Autodesk Inventor part; units mm, degrees
ref_plane "YZ Plane" through (0, 0, 0) normal (1, 0, 0) x (0, 1, 0)
ref_plane "XZ Plane" through (0, 0, 0) normal (0, 1, 0) x (-1, 0, 0)
ref_plane "XY Plane" through (0, 0, 0) normal (0, 0, 1) x (1, 0, 0)
sketch "スケッチ1" plane through (0, 0, 0) normal (0, 0, 1) x (1, 0, 0)
  circle A0 centre (0, 0) radius 23
  dimension "d0" = 46
extrude "押し出し1" add sketch "スケッチ1" along normal blind 6.3
sketch "スケッチ2" plane through (0, 0, 6.3) normal (0, 0, 1) x (1, 0, 0)
  line L0 (0, 0) -> (16.85, 0)
  line L1 (16.85, 0) -> (16.85, 13.85)
  line L2 (16.85, 13.85) -> (0, 13.85)
  line L3 (0, 13.85) -> (0, 0)
  line L4 (0, 0) -> (-16.85, 0)
  line L5 (-16.85, 0) -> (-16.85, 13.85)
  line L6 (-16.85, 13.85) -> (0, 13.85)
  line L7 (-19.95, -13.85) -> (19.95, -13.85)
  line L8 (19.95, -13.85) -> (19.95, 16.85)
  line L9 (19.95, 16.85) -> (-19.95, 16.85)
  line L10 (-19.95, 16.85) -> (-19.95, -13.85)
  line L11 (-16.85, 0) -> (-16.85, -13.85)
  line L12 (16.85, 0) -> (16.85, -13.85)
  circle A0 centre (0, 0) radius 23
  point P0 (18.3624, -13.85)
  point P1 (19.95, -11.4454)
  point P2 (19.95, 11.4454)
  point P3 (15.655, 16.85)
  point P4 (-15.655, 16.85)
  point P5 (-19.95, 11.4454)
  point P6 (-19.95, -11.4454)
  point P7 (-18.3624, -13.85)
  dimension "d3" = 13.85
  dimension "d4" = 16.85
  dimension "d5" = 3
  dimension "d6" = 3.1
  dimension "d8" = 3.1
  dimension "d9" = 30.7
  dimension "d10" = 46
extrude "押し出し2" add sketch "スケッチ2" along normal blind 5.6 contours L1 L2 L6 L5 L11 L7 A0 L10 L9 L8 L12
sketch "スケッチ3" plane through (0, 0, 6.3) normal (0, 0, 1) x (1, 0, 0)
  circle A0 centre (0, 0) radius 13.1
  dimension "d13" = 26.2
extrude "押し出し3" cut sketch "スケッチ3" against normal blind 7
sketch "スケッチ4" plane through (0, 0, 0) normal (0, 0, -1) x (-1, 0, 0)
  circle A0 centre (0, 0) radius 19.5
  dimension "d16" = 39
extrude "押し出し4" [suppressed]
fillet "フィレット1" radius 1 3 edges at (0, 16.85, 6.3) (19.95, 0, 6.3) (-19.95, 0, 6.3)
properties part number "connectpart2"
The listing builds one solid part. Answer for the finished solid, in the listing's coordinates (mm). A direction names the side the tool comes from. Give positions to 0.01 mm unless a question says otherwise; leave off trailing zeros. Write each loop counter-clockwise with the first axis right and the second up, starting at its lowest first coordinate (ties: lowest second). Pieces come first, ordered by that corner, then holes.
1) Section B-B (x = 0) is taken. Write down the section's boundary in (y, z), and give its area (3 significant figures).
2) Section C-C (z = 4) is taken. Write down the section's boundary in (x, y).
3) Find the intervals of material crossed by L1, parallel to Y at x = 0, z = 4; L2, parallel to X at y = 0, z = 10.75; L3, parallel to Z at x = 4, y = -13, in increasing order.
4) Section D-D (x = -12.5) is taken. Write down the section's boundary in (y, z), and give its area (3 significant figures).
5) Section A-A (y = 0) is taken. Write down the section's boundary in (x, z), and give its area (3 significant figures).
6) A tool of negligible diameter and unlimited length cuts with its end or side. For faces 5 (the face through (-19.95, 0, 10)), 6 (the face through (0, 13.85, 9)), 7 (the face through (22, 0, 6.3)), 8 (the face through (18, -13.85, 9)), from which of +Z, -Z, +X, -X, +Y, -Y can it reach the whole face along a straight path? Write none if from no direction.
7) For a pull along Y with two mould halves and no side action, classify faces 1 (the face through (-18, -13.85, 9)), 2 (the face through (0, 16.85, 10)), 3 (the face through (-1.705, 12.989, 3.194)), 4 (the face through (-22, 0, 6.3)) as pulls with the +Y half, pulls with the -Y half, needs draft (parallel to the pull), parting line crosses it, or undercut.
8) Given P1, Ø4, axis at x = 5.5, y = 19.5, coming from the +Z side; P2, Ø3, axis at y = -0.5, z = 9.5, coming from the -X side; P3, Ø1.7, axis at x = -18, z = 8.5, coming from the -Y side, each flat-ended and moving along its own axis, determine where each tip first touches the part or whether it passes through.
Response:
1. outline: (-23, 0) - (-13.1, 0) - (-13.1, 6.3) - (-23, 6.3) - close; (13.1, 0) - (23, 0) - (23, 6.3) - (17.85, 6.3) arc R1 cw to (16.85, 7.3) - (16.85, 11.9) - (13.85, 11.9) - (13.85, 6.3) - (13.1, 6.3) - close
1. area: 142 mm2
2. outline: circle Ø46 at (0, 0); hole circle Ø26.2 at (0, 0)
3. L1: y = -23 to -13.1, 13.1 to 23
3. L2: x = -19.95 to -16.85, 16.85 to 19.95
3. L3: z = 0 to 6.3
4. outline: (-19.31, 0) - (-3.92, 0) - (-3.92, 6.3) - (-19.31, 6.3) - close; (3.92, 0) - (19.31, 0) - (19.31, 6.3) - (17.85, 6.3) arc R1 cw to (16.85, 7.3) - (16.85, 11.9) - (13.85, 11.9) - (13.85, 6.3) - (3.92, 6.3) - close
4. area: 211 mm2
5. outline: (-23, 0) - (-13.1, 0) - (-13.1, 6.3) - (-16.85, 6.3) - (-16.85, 11.9) - (-19.95, 11.9) - (-19.95, 7.3) arc R1 cw to (-20.95, 6.3) - (-23, 6.3) - close; (13.1, 0) - (23, 0) - (23, 6.3) - (20.95, 6.3) arc R1 cw to (19.95, 7.3) - (19.95, 11.9) - (16.85, 11.9) - (16.85, 6.3) - (13.1, 6.3) - close
5. area: 160 mm2
6. face 5: +Z, -X, +Y, -Y
6. face 6: +Z, -Y
6. face 7: +Z, +X, +Y, -Y
6. face 8: +Z, +X, -X, -Y
7. face 1: pulls with the -Y half
7. face 2: pulls with the +Y half
7. face 3: undercut
7. face 4: needs draft
8. P1: stops at z = 6.36
8. P2: stops at x = -19.95
8. P3: stops at y = -13.85
